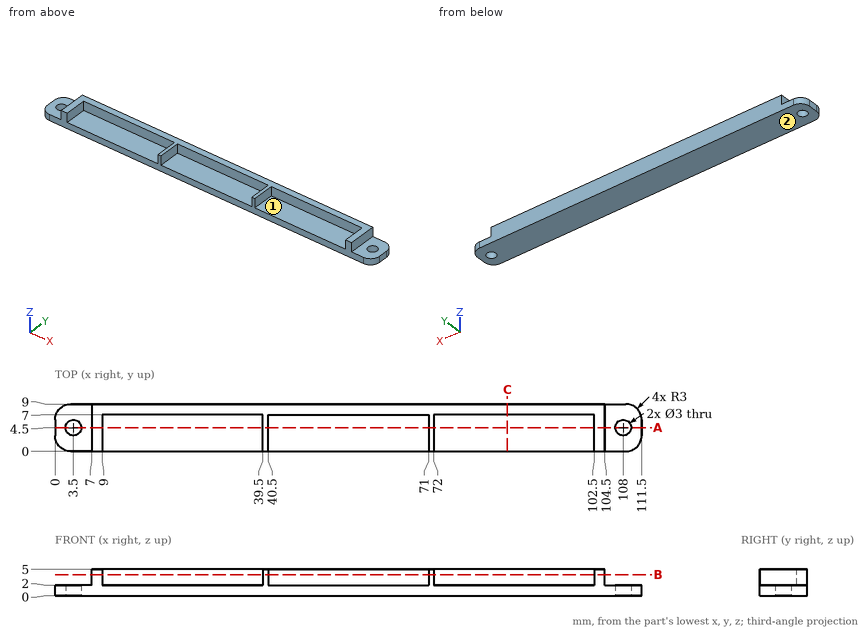
The figure shows three views and two pictorial views of one solid part (mm, origin at its lowest corner). Answer the questions. Coordinates: 2 decimals unless noted, no trailing zeros. Loops run counter-clockwise (first coordinate to the right, second up) from the corner with the lowest first, then second, coordinate; pieces in that order, holes last. Notation, with made-up numbers: (-4, 60) - (41, 60) arc R25 ccw to (41, 82) - close; hole circle Ø7 at (-11, 42.5). An arc over 180 degrees is marked (long way). Use a Markdown table: item, result. Add a question column.
1) The part is cut by section A-A, the plane y = 4.5. Give the vertices of the cut face in (x, z), and give its area (3 significant figures).
2) The mould has two halves that part along X. Classify the marked faces 1 and 2: released by +X, released by -X, zero draft, split by the parting line, or undercut.
3) The part is cut by section C-C, the plane x = 86. Give the vertices of the cut face in (y, z), and give its area (3 significant figures).
4) The part is cut by section B-B, the plane z = 4. Give the vertices of the cut face in (x, y), and give its area (3 significant figures).
5) Given pin 1 (0.9 mm diameter, centred on y = 3.5, z = 4, fed in from +X); pin 2 (2 mm diameter, centred on x = 107, y = 4, fed in from +Z); pin 3 (0.9 mm diameter, centred on y = 2.5, z = 3.5, fed in from -X), each flat-ended and moving along its own axis, determine where each tip first touches the part or whether it passes through.
6) Find the intervals of material crossed by line 1 (X direction, y = 4.5, z = 1.2); line 2 (X direction, y = 3, z = 2.2); line 3 (Y direction, x = 3.5, z = 0.8), in increasing order.
Here are the results:
| question | item | result |
|---|---|---|
| 1 | outline | (0, 0) - (2, 0) - (2, 2) - (0, 2) - close; (5, 0) - (106.5, 0) - (106.5, 2) - (104.5, 2) - (104.5, 5) - (102.5, 5) - (102.5, 2) - (72, 2) - (72, 5) - (71, 5) - (71, 2) - (40.5, 2) - (40.5, 5) - (39.5, 5) - (39.5, 2) - (9, 2) - (9, 5) - (7, 5) - (7, 2) - (5, 2) - close; (109.5, 0) - (111.5, 0) - (111.5, 2) - (109.5, 2) - close |
| 1 | area | 229 mm^2 |
| 2 | face 1 | undercut |
| 2 | face 2 | zero draft |
| 3 | outline | (0, 0) - (9, 0) - (9, 5) - (7, 5) - (7, 2) - (0, 2) - close |
| 3 | area | 24.0 mm^2 |
| 4 | outline | (7, 0) - (9, 0) - (9, 7) - (39.5, 7) - (39.5, 0) - (40.5, 0) - (40.5, 7) - (71, 7) - (71, 0) - (72, 0) - (72, 7) - (102.5, 7) - (102.5, 0) - (104.5, 0) - (104.5, 9) - (7, 9) - close |
| 4 | area | 237 mm^2 |
| 5 | pin 1 | stops at x = 104.5 |
| 5 | pin 2 | stops at z = 2 |
| 5 | pin 3 | stops at x = 7 |
| 6 | line 1 | x = 0 to 2, 5 to 106.5, 109.5 to 111.5 |
| 6 | line 2 | x = 7 to 9, 39.5 to 40.5, 71 to 72, 102.5 to 104.5 |
| 6 | line 3 | y = 0 to 3, 6 to 9 |
